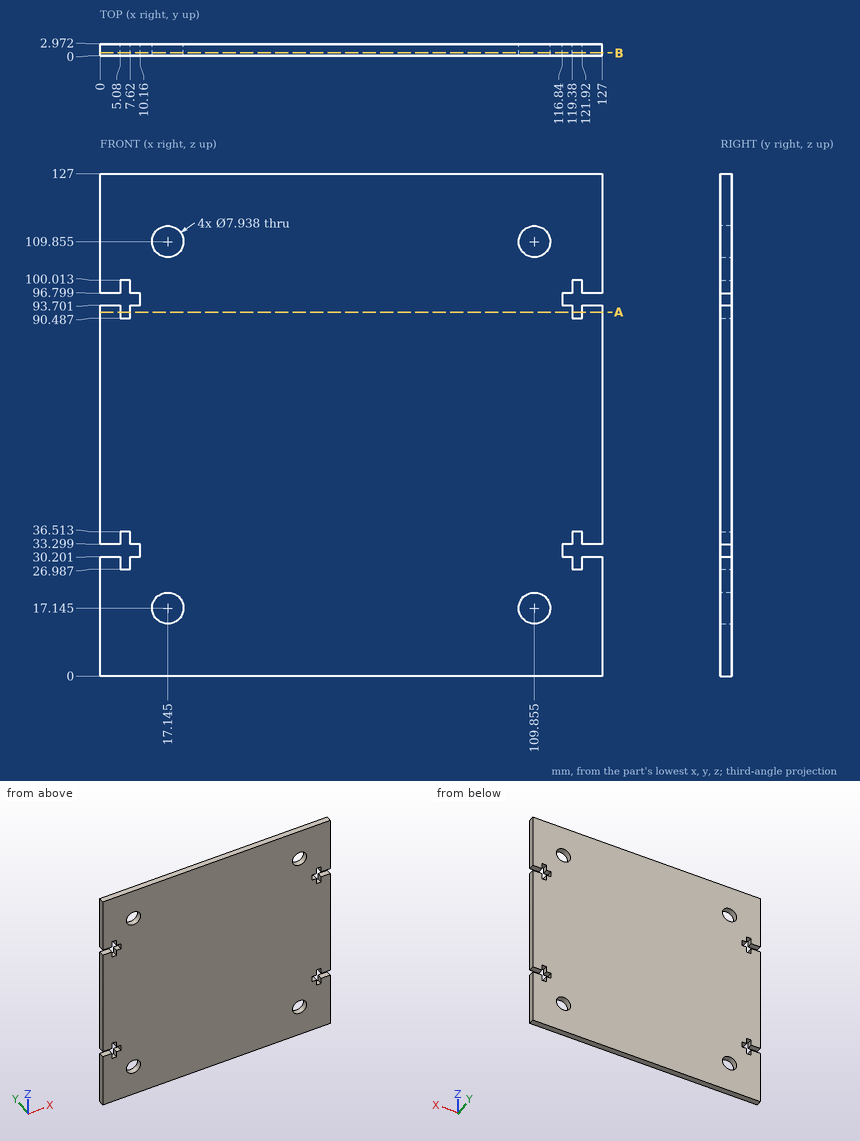
For this review, use the dimensioned drawing (mm, ordinates from the lowest corner) and the shaded views. Coordinates: 2 decimals unless noted, no trailing zeros. Order: outer loops, then holes, each group sorted by start corner. A loop starts at its lowest first (then second) coordinate and runs counter-clockwise, first axis right, second up. Notation, with made-up numbers: (63.5, 63.25) - (119.5, 63.25) arc R16 cw to (119.5, 77.25) - close; hole circle Ø7 at (9, -0.5). An arc over 180 degrees is marked (long way). Answer as a JSON object with one key per item and string values. Group by question number.
1. We need section A-A on z = 92. State the section outline as (x, y) points.
2. We need section B-B on y = 0.7. Give the number of separate pieces and of enclosed holes in the cut face, then the cut area to 3 significant figures.
3. For probe 1 along Z at (x, y) = (119, 0.55); probe 2 along Z at (x, y) = (109, 2), list the stretches that pass through material, from the lowest coordinate up.
4. Clearance check with flat-ended pins moving along their axes: P1, Ø0.9, axis at y = 1.5, z = 92.5, coming from the -X side; P2, Ø5, axis at x = 109.855, z = 109.855, coming from the -Y side. State where each tip first meets the part, or that it passes through.
Final values:
{
 "1": {"outline": "(0, 0) - (5.08, 0) - (5.08, 2.97) - (0, 2.97) - close; (7.62, 0) - (119.38, 0) - (119.38, 2.97) - (7.62, 2.97) - close; (121.92, 0) - (127, 0) - (127, 2.97) - (121.92, 2.97) - close"},
 "2": {"separate pieces": "1", "enclosed holes": "4", "area": "15,700 mm²"},
 "3": {"probe 1": "0 to 30.2, 33.3 to 93.7, 96.8 to 127", "probe 2": "0 to 13.27, 21.02 to 105.98, 113.73 to 127"},
 "4": {"P1": "x = 0", "P2": "through"}
}
